from build123d import *
from OCP.BRepFilletAPI import BRepFilletAPI_MakeChamfer

# Parameters (mm, degrees)
SCHIZZO1_R                   = 1.75
ESTRUSIONE_ESTRUSIONE1_DEPTH = 2
SMUSSO1_SIZE                 = 20
SMUSSO1_SIZE2                = 28.562960135
TAGLIO_ESTRUSIONE1_DEPTH     = 10
RACCORDO1_R                  = 10
RACCORDO2_R                  = 20


with BuildPart() as part:
    # Schizzo1 → Estrusione-Estrusione1 (new body)
    with BuildSketch(Plane(origin=(0, 0, 0), x_dir=(1, 0, 0), z_dir=(0, 1, 0))):
        Polygon((-10, -57.5), (-10, -100), (10, -100), (10, -57.5), (17.5, -57.5), (17.5, -42.5), (10, -42.5), (10, 12.5), (55, 12.5), (55, 100), (10, 100), (-10, 100), (-30, 100), (-30, 12.5), (-10, 12.5), (-10, -42.5), (-17.5, -42.5), (-17.5, -57.5), align=None)
        with Locations(Location((0, -87.75, 0), (0, 0, 270))):
            Circle(SCHIZZO1_R, mode=Mode.SUBTRACT)
        with Locations(Location((0, -62.75, 0), (0, 0, 270))):
            Circle(SCHIZZO1_R, mode=Mode.SUBTRACT)
        with Locations(Location((-12, -50, 0), (0, 0, 270))):
            Circle(SCHIZZO1_R, mode=Mode.SUBTRACT)
        with Locations(Location((0, -37.75, 0), (0, 0, 270))):
            Circle(SCHIZZO1_R, mode=Mode.SUBTRACT)
        with Locations(Location((12, -50, 0), (0, 0, 270))):
            Circle(SCHIZZO1_R, mode=Mode.SUBTRACT)
        with Locations(Location((0, -12.75, 0), (0, 0, 270))):
            Circle(SCHIZZO1_R, mode=Mode.SUBTRACT)
        with Locations(Location((-12, 56.25, 0), (0, 0, 270))):
            Circle(SCHIZZO1_R, mode=Mode.SUBTRACT)
        with Locations(Location((12, 56.25, 0), (0, 0, 270))):
            Circle(SCHIZZO1_R, mode=Mode.SUBTRACT)
        with Locations(Location((25.04, 26.25, 0), (0, 0, 270))):
            Circle(SCHIZZO1_R, mode=Mode.SUBTRACT)
        with Locations(Location((25.04, 86.25, 0), (0, 0, 270))):
            Circle(SCHIZZO1_R, mode=Mode.SUBTRACT)
        with Locations(Location((47.2, 56.25, 0), (0, 0, 270))):
            Circle(SCHIZZO1_R, mode=Mode.SUBTRACT)
    extrude(amount=-ESTRUSIONE_ESTRUSIONE1_DEPTH)

    # Smusso1: one chamfer whose edges measure the first distance from different faces: ONE call of the kernel's chamfer builder (chamfer() names one face for all edges)
    smusso1_edges_1 = [part.edges().sort_by_distance(p)[0] for p in [
        (55, -1, -12.5),
    ]]
    smusso1_side_1 = [part.faces().sort_by_distance(p)[0] for p in [
        (32.5, -1, -12.5),
    ]]
    smusso1_edges_2 = [part.edges().sort_by_distance(p)[0] for p in [
        (55, -1, -100),
    ]]
    smusso1_side_2 = [part.faces().sort_by_distance(p)[0] for p in [
        (12.5, -1, -100),
    ]]
    smusso1 = BRepFilletAPI_MakeChamfer(part.part.solid().wrapped)
    for e in smusso1_edges_1:
        smusso1.Add(SMUSSO1_SIZE, SMUSSO1_SIZE2, e.wrapped, smusso1_side_1[0].wrapped)  # the first distance lies on this face
    for e in smusso1_edges_2:
        smusso1.Add(SMUSSO1_SIZE, SMUSSO1_SIZE2, e.wrapped, smusso1_side_2[0].wrapped)  # the first distance lies on this face
    add(Compound.cast(smusso1.Shape()), mode=Mode.REPLACE)

    # Schizzo2 → Taglio-Estrusione1 (cut)
    with BuildSketch(Plane(origin=(0, 0, 0), x_dir=(1, 0, 0), z_dir=(0, 1, 0))):
        Polygon((-10, 12.5), (-10, 48.75), (-17.5, 48.75), (-17.5, 63.75), (-10.178518111, 63.75), (-10.178518111, 100), (-33.809151811, 100), (-33.809151811, 12.5), align=None)
    extrude(amount=-TAGLIO_ESTRUSIONE1_DEPTH, mode=Mode.SUBTRACT)

    # Raccordo1
    # the kernel refuses this fillet: 10 mm, written as the material it adds along each edge
    with BuildSketch(Plane(origin=(10, 0, 42.5), x_dir=(0, 0, -1), z_dir=(0, -1, 0)), Plane(origin=(-10, 0, 57.5), x_dir=(0, 0, 1), z_dir=(0, -1, 0)), Plane(origin=(-10, 0, -48.75), x_dir=(0, 0, 1), z_dir=(0, -1, 0))) as raccordo1_piece_1:
        with BuildLine():
            CenterArc((9.682458366, 10), RACCORDO1_R, 194.477512186, 75.522487814)
            Line((0, 7.5), (0, 0))
            Line((0, 0), (9.682458366, 0))
        make_face()
    extrude(amount=2)
    with BuildSketch(Plane(origin=(-10, 0, 42.5), x_dir=(-1, 0, 0), z_dir=(0, -1, 0)), Plane(origin=(10, 0, 57.5), x_dir=(1, 0, 0), z_dir=(0, -1, 0))) as raccordo1_piece_2:
        with BuildLine():
            CenterArc((10, 9.682458366), RACCORDO1_R, 180, 75.522487814)
            Line((0, 9.682458366), (0, 0))
            Line((0, 0), (7.5, 0))
        make_face()
    extrude(amount=2)
    with BuildSketch(Plane(origin=(-10.178518111, 0, -63.75), x_dir=(-1, 0, 0), z_dir=(0, -1, 0))) as raccordo1_piece_3:
        with BuildLine():
            CenterArc((10, 9.634601223), RACCORDO1_R, 180, 74.463523002)
            Line((0, 9.634601223), (0, 0))
            Line((0, 0), (7.321481889, 0))
        make_face()
    extrude(amount=2)
    # the kernel refuses this fillet: 10 mm, written as the material it takes off along each edge
    with BuildSketch(Plane(origin=(35, 13.014176264, -12.5), x_dir=(-1, 0, 0), z_dir=(0, -1, 0)), Plane(origin=(35, 13.014176264, -100), x_dir=(0.5735764363510455, 0, 0.8191520442889922), z_dir=(0, -1, 0))) as raccordo1_2_piece_1:
        with BuildLine():
            CenterArc((RACCORDO1_R * 0.520567050552, RACCORDO1_R), RACCORDO1_R, 215, 55)
            Line((-RACCORDO1_R * 0.298584993737, RACCORDO1_R * 0.426423563649), (0, 0))
            Line((0, 0), (RACCORDO1_R * 0.520567050552, 0))
        make_face()
    extrude(amount=28.028352528, mode=Mode.SUBTRACT)
    with BuildSketch(Plane(origin=(55, 7.882469722, -41.062960135), x_dir=(-0.5735764363510429, 0, 0.819152044288994), z_dir=(0, -1, 0)), Plane(origin=(55, 7.882469722, -71.437039865), x_dir=(0, 0, 1), z_dir=(0, -1, 0))) as raccordo1_2_piece_2:
        with BuildLine():
            CenterArc((RACCORDO1_R * 0.315298788879, RACCORDO1_R), RACCORDO1_R, 235, 35)
            Line((-RACCORDO1_R * 0.258277647472, RACCORDO1_R * 0.180847955711), (0, 0))
            Line((0, 0), (RACCORDO1_R * 0.315298788879, 0))
        make_face()
    extrude(amount=17.764939444, mode=Mode.SUBTRACT)
    with BuildSketch(Plane(origin=(-10.178518111, 25, -100), x_dir=(1, 0, 0), z_dir=(0, -1, 0))) as raccordo1_2_piece_3:
        with BuildLine():
            CenterArc((RACCORDO1_R, RACCORDO1_R), RACCORDO1_R, 180, 90)
            Line((0, RACCORDO1_R), (0, 0))
            Line((0, 0), (RACCORDO1_R, 0))
        make_face()
    extrude(amount=52, mode=Mode.SUBTRACT)

    # Raccordo2
    raccordo2_edges = [part.edges().sort_by_distance(p)[0] for p in [
        (10, -1, -12.5),
    ]]
    fillet(raccordo2_edges, radius=RACCORDO2_R)


solid = part.part
Part model, mm, in its own coordinate system. A direction names the side the tool comes from. Round coordinates to 2 decimals unless told otherwise and drop trailing zeros. Order: outer loops, then holes, each group sorted by start corner. A loop starts at its lowest first (then second) coordinate and runs counter-clockwise, first axis right, second up. Notation, with made-up numbers: (-18, -9) -> (17, -9) arc R33 cw to (17, 27) -> close; hole circle Ø7 at (-24, 89.25). An arc over 180 degrees is marked (long way). Put each result on its own line as item: value.
Q1. Pull direction X, two halves, no side cores. Call faces 1 (the face through (12.526, -0.986, -54.581)), 2 (the face through (10, 0, -24)), 3 (the face through (45.695, -0.986, -27.774)): pulls with the +X half, pulls with the -X half, needs draft (parallel to the pull), parting line crosses it, or undercut.
From the geometry:
face 1: undercut
face 2: needs draft
face 3: pulls with the +X half
Q2. Tool access for faces 4 (the face through (-12.04, -0.99, 38.87)), 5 (the face through (47.726, -0.986, -54.581)), 6 (the face through (12.15, -0.99, 39.01)): list every direction of +Z, -Z, +X, -X, +Y, -Y with a clear straight run to the whole face (end or side of a thin tool).
From the geometry:
face 4: -X, +Y, -Y
face 5: +Y, -Y
face 6: +X, +Y, -Y
Q3. Pin check, flat tip, straight feed: pin 1 Ø3 at (x, z) = (0, 12.75) entering from -Y. Stop position of the tip, or through.
From the geometry:
pin 1: passes through
Q4. Band-saw the part on D-D (z = 80.5). Give the cut face in (x, y).
From the geometry:
outline: (-10, -2) -> (10, -2) -> (10, 0) -> (-10, 0) -> close
Q5. Band-saw the part on C-C (x = -12). Give the cut face in (y, z), and give its area (3 significant figures).
From the geometry:
outline: (-2, -67.63) -> (0, -67.63) -> (0, -58) -> (-2, -58) -> close; (-2, -54.5) -> (0, -54.5) -> (0, -45.07) -> (-2, -45.07) -> close; (-2, 38.82) -> (0, 38.82) -> (0, 48.25) -> (-2, 48.25) -> close; (-2, 51.75) -> (0, 51.75) -> (0, 61.18) -> (-2, 61.18) -> close
area: 75.9 mm2
Q6. Wall check: line 1 (X direction, y = -0.9, z = 87.75); line 2 (Z direction, x = 1.5, y = -1.05); line 3 (X direction, y = -0.5, z = 83). Give the ranges that are in metal, low to high. Write a range as [from, to].
From the geometry:
line 1: x = [-10, -1.75], [1.75, 10]
line 2: z = [-100, 11.85], [13.65, 36.85], [38.65, 61.85], [63.65, 86.85], [88.65, 100]
line 3: x = [-10, 10]
Q7. Band-saw the part on B-B (z = 37.75). Give the cut face in (x, y), and give its area (3 significant figures).
From the geometry:
outline: (-11.3, -2) -> (-1.75, -2) -> (-1.75, 0) -> (-11.3, 0) -> close; (1.75, -2) -> (11.3, -2) -> (11.3, 0) -> (1.75, 0) -> close
area: 38.2 mm2
Q8. Band-saw the part on A-A (x = 47.2). Give the cut face in (y, z), and give its area (3 significant figures).
From the geometry:
outline: (-2, -82.58) -> (0, -82.58) -> (0, -58) -> (-2, -58) -> close; (-2, -54.5) -> (0, -54.5) -> (0, -29.92) -> (-2, -29.92) -> close
area: 98.3 mm2
